Part model, mm, in its own coordinate system. Face numbers are marked on the shaded views. A direction names the side the tool comes from. Coordinates: 2 decimals unless noted, no trailing zeros. Loops run counter-clockwise (first coordinate to the right, second up) from the corner with the lowest first, then second, coordinate; pieces in that order, holes last. Notation, with made-up numbers: (-1.75, 67.25) -> (43.25, 67.25) arc R18 cw to (43.25, 90.25) -> close; hole circle Ø5 at (50.5, -20.5). An arc over 180 degrees is marked (long way). One line per question, with ' | ' between items. Start each with the question number.
1) Probe L1, parallel to X at y = 0, z = 2.95; L2, parallel to Z at x = -6.5, y = 7.25. List the from-to ranges inside material, lowest first. Write a range as from..to.
2) Cut at D-D (z = 3.75). List the corners of the cut face in (x, y), plus the area to 3 significant figures.
3) Two-plate mould, pull along Y, no slides. Class the marked faces 1, 2 and 3: released by +Y, released by -Y, zero draft, split by the parting line, or undercut.
4) Drop flat-ended pins along their axis: pin 1 (4 mm diameter, centred on y = 4, z = 8, fed in from -X); pin 2 (3 mm diameter, centred on x = -7.5, z = 6, fed in from -Y); pin 3 (8 mm diameter, centred on x = -2, y = -0.5, fed in from +Z); pin 4 (1.5 mm diameter, centred on x = -7, z = 7, fed in from +Y). Give the stop position or say it passes through.
5) Cut at C-C (x = 0). List the corners of the cut face in (y, z).
6) 3-axis set-ups, long thin cutter, end or side, ignore diameter. For the marked faces 4, 5, 6 and 7: which of +Z, -Z, +X, -X, +Y, -Y reach the whole face in a straight line?
7) Cut at B-B (y = -3.5). List the corners of the cut face in (x, z).
8) Cut at A-A (z = 5.25). List the corners of the cut face in (x, y), plus the area to 3 significant figures.
from build123d import *
from build123d import SkipClean  # not in build123d's __all__

# Parameters (mm, degrees)
F0_R     = 10
F0_R_2   = 5
F1_DEPTH = 5
F3_DEPTH = 5


with BuildPart() as f1:
    # F0 (on Top) → F1 (new body)
    with BuildSketch(Plane.XY):
        Circle(F0_R)
        Circle(F0_R_2, mode=Mode.SUBTRACT)
    extrude(amount=F1_DEPTH)

    # F2 (on face) → F3 (join)
    with BuildSketch(Plane.XY.offset(5)):
        with BuildLine():
            ThreePointArc((-2.5, -4.3301270189), (-4.3301270189, -2.5), (-5, 0))
            Line((-5, 0), (-10, 0))
            ThreePointArc((-10, 0), (-8.6602540378, -5), (-5, -8.6602540378))
            Line((-5, -8.6602540378), (-2.5, -4.3301270189))
        make_face()
        with BuildLine():
            ThreePointArc((5, 0), (4.3301270189, -2.5), (2.5, -4.3301270189))
            Line((2.5, -4.3301270189), (5, -8.6602540378))
            ThreePointArc((5, -8.6602540378), (8.6602540378, -5), (10, 0))
            Line((10, 0), (5, 0))
        make_face()
        with BuildLine():
            ThreePointArc((-2.5, 4.3301270189), (0, 5), (2.5, 4.3301270189))
            Line((2.5, 4.3301270189), (5, 8.6602540378))
            ThreePointArc((5, 8.6602540378), (0, 10), (-5, 8.6602540378))
            Line((-5, 8.6602540378), (-2.5, 4.3301270189))
        make_face()
    with SkipClean():  # cleaning this boolean's faces spoils the solid; the shape is the same uncleaned
        extrude(amount=F3_DEPTH)


solid = f1.part
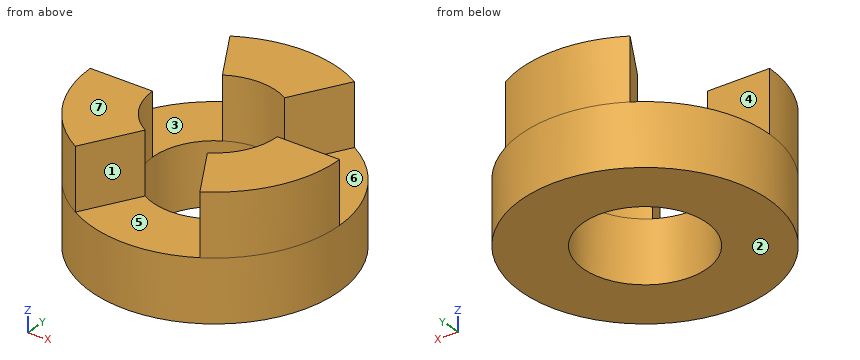
Reported:
1) L1: x = -10..-5, 5..10 | L2: z = 0..5
2) outline: circle Ø20 at (0, 0); hole circle Ø10 at (0, 0) | area: 236 mm²
3) face 1: released by -Y | face 2: zero draft | face 3: undercut
4) pin 1: stops at x = -3.46 | pin 2: stops at y = -8 | pin 3: stops at z = 10 | pin 4: stops at y = 0
5) outline: (-10, 0) -> (-5, 0) -> (-5, 5) -> (-10, 5) -> close; (5, 0) -> (10, 0) -> (10, 10) -> (5, 10) -> close
6) face 4: +Z, +X, -X, +Y | face 5: +Z, -Y | face 6: +Z, +X | face 7: +Z, +X, -X, +Y, -Y
7) outline: (-9.37, 0) -> (-3.57, 0) -> (-3.57, 10) -> (-9.37, 10) -> close; (3.57, 0) -> (9.37, 0) -> (9.37, 10) -> (3.57, 10) -> close
8) outline: (-10, 0) arc R10 ccw to (-5, -8.66) -> (-2.5, -4.33) arc R5 cw to (-5, 0) -> close; (-5, 8.66) -> (-2.5, 4.33) arc R5 cw to (2.5, 4.33) -> (5, 8.66) arc R10 ccw to start; (2.5, -4.33) -> (5, -8.66) arc R10 ccw to (10, 0) -> (5, 0) arc R5 cw to start | area: 118 mm²
